Autodesk Inventor part; units mm, degrees
ref_plane "YZ Plane" through (0, 0, 0) normal (1, 0, 0) x (0, 1, 0)
ref_plane "XZ Plane" through (0, 0, 0) normal (0, 1, 0) x (-1, 0, 0)
ref_plane "XY Plane" through (0, 0, 0) normal (0, 0, 1) x (1, 0, 0)
sketch "Boceto1" plane through (0, 0, 0) normal (0, 1, 0) x (-1, 0, 0)
  line L0 (0, 0) -> (-45, 0)
  line L1 (-45, 0) -> (-45, -19)
  line L2 (-45, -19) -> (0, -19)
  line L3 (0, -19) -> (0, 0)
extrude "Extrusión1" add sketch "Boceto1" along normal blind 19.5
sketch "Boceto2" plane through (0, 19.5, 0) normal (0, 1, 0) x (1, 0, 0)
  line L0 (0, 19) -> (0, 0)
  line L1 (45, 0) -> (45, 19)
  line L2 (0, 0) -> (45, 0)
  line L3 (45, 19) -> (0, 19)
  line L4 (0.3, 0.3) -> (0.3, 9.5)
  line L5 (0.3, 0.3) -> (12.3526, 0.3)
  line L6 (0.3, 9.5) -> (0.3, 18.7)
  line L7 (0.3, 18.7) -> (13.3767, 18.7)
  line L8 (13.3767, 18.7) -> (25.3714, 18.7)
  line L9 (25.3714, 18.7) -> (38.8857, 18.7)
  line L10 (44.7, 0.3) -> (44.7, 18.7)
  line L11 (44.7, 18.7) -> (38.8857, 18.7)
  line L12 (44.7, 0.3) -> (33.7568, 0.3)
  line L13 (12.3526, 0.3) -> (33.7568, 0.3)
extrude "Extrusión2" cut sketch "Boceto2" against normal blind 19 contours L4 L6 L7 L8 L9 L11 L10 L12 L13 L5
equation "\"Radio_pliegue\" = Grosor"
equation "\"Anchura_desahogo_plegado\" = Grosor"
equation "\"Profundidad_desahogo_plegado\" = 0.5 * Grosor"
equation "\"Tamaño_destalonado\" = 4 * Grosor"
equation "\"Remanente_mínimo\" = 2 * Grosor"
equation "\"Radiodetransición\" = Radio_pliegue"
equation "\"Tamaño_de_radio_de_Jacobi\" = Radio_pliegue"
equation "\"TamañoSeparación\" = Grosor"
properties part number "caja"
Check sheet for the modelled part. Datum: model origin and axes. Units: mm. A direction names the side the tool comes from. Give positions to 0.01 mm unless a question says otherwise; leave off trailing zeros. Write each loop counter-clockwise with the first axis right and the second up, starting at its lowest first coordinate (ties: lowest second). Pieces come first, ordered by that corner, then holes.
Item 1: Cross-section at C-C (z = -3). Enter the section's corners in (x, y), and give its area (3 significant figures).
Item 2: Cross-section at B-B (x = 19). Enter the section's corners in (y, z).
Item 3: Scan lines: L1, parallel to Z at x = 29, y = 1.75; L2, parallel to X at y = 5.75, z = -14.5; L3, parallel to Y at x = 32, z = -9.25. Record each from-to range of solid material in increasing order.
Item 4: Cross-section at A-A (y = 10.25). Enter the section's corners in (x, z), and give its area (3 significant figures).
Item 5: Gauge pin test, flat end, axial feed: pin 1 (2 mm diameter, centred on x = 23.5, z = -5.5, fed in from +Y). Record the tip position at first contact, or that the pin passes through.
Item 6: Access from +Z, -Z, +X, -X, +Y, -Y to the whole of each face (thin tool, end or side, straight path). Record for faces 4 (the face through (44.7, 10, -9)), 5 (the face through (23, 10, -19)).
Item 7: Draft check along Z on faces 1 (the face through (22, 10, 0)), 2 (the face through (23, 10, -18.7)), 3 (the face through (45, 10, -9)). Enter one of: released by +Z, released by -Z, zero draft, split by the parting line, or undercut.
Report:
1. outline: (0, 0) - (45, 0) - (45, 19.5) - (44.7, 19.5) - (44.7, 0.5) - (0.3, 0.5) - (0.3, 19.5) - (0, 19.5) - close
1. area: 33.9 mm2
2. outline: (0, -19) - (19.5, -19) - (19.5, -18.7) - (0.5, -18.7) - (0.5, -0.3) - (19.5, -0.3) - (19.5, 0) - (0, 0) - close
3. L1: z = -19 to -18.7, -0.3 to 0
3. L2: x = 0 to 0.3, 44.7 to 45
3. L3: y = 0 to 0.5
4. outline: (0, -19) - (45, -19) - (45, 0) - (0, 0) - close; hole (0.3, -18.7) - (44.7, -18.7) - (44.7, -0.3) - (0.3, -0.3) - close
4. area: 38.0 mm2
5. pin 1: stops at y = 0.5
6. face 4: +Y
6. face 5: -Z, +X, -X, +Y, -Y
7. face 1: released by +Z
7. face 2: undercut
7. face 3: zero draft
